Can you work these out from the model? Positions are in its coordinate system, mm. A direction names the side the tool comes from. Give positions to 0.01 mm unless a question says otherwise; leave off trailing zeros. Order: outer loops, then holes, each group sorted by start corner. A loop starts at its lowest first (then second) coordinate and runs counter-clockwise, first axis right, second up.
Item 1: I want a section at C-C, the plane y = 13. Write out the boundary of the cut face in (x, z), then the cut area to 3 significant figures.
Item 2: Which directions (+Z, -Z, +X, -X, +Y, -Y) give clear straight access to the entire face, cutting with the end or side of a thin tool? Please do faces 1 (the flat face through (-53.272, 10, 1)), 2 (the flat face through (38.836, 9.86, 25.136)), 3 (the flat face through (40.712, 9.86, 19.134)), 4 (the flat face through (37.063, 10, -23)).
Item 3: I'm going to push flat-ended pins straight in: pin 1 Ø3 at (y, z) = (12.5, -13.5) entering from -X; pin 2 Ø1.5 at (y, z) = (8.5, 11) entering from +X; pin 3 Ø5 at (y, z) = (9, 20.5) entering from +X. Where does each tip first touch, or does it pass through?
Item 4: If I drill on line 1 along Z through (x, y) = (42, 8.75); line 2 along Z through (x, y) = (41.5, 3); line 3 along X through (y, z) = (8.25, -2), over which ranges is the centre line in solid material (lowest first)?
Item 5: I want a section at B-B, the plane z = -20.5. Write out the boundary of the cut face in (x, y), then the cut area to 3 significant figures.
Item 6: If we mould it in two halves opening along Z, with no side actions, what happens to faces 5 (the flat face through (-11, 10, -27.075)), 6 (the cylindrical face through (43.73, 3.56, -19.28)), 7 (the flat face through (-58.473, 10, 24))? For each: +Z half, -Z half, draft (parallel to the pull), parting line (faces both ways), or undercut.
Item 7: I want a section at D-D, the plane z = -14. Write out the boundary of the cut face in (x, y), then the cut area to 3 significant figures.
Item 8: I want a section at A-A, the plane y = 6.5. Write out the boundary of the cut face in (x, z).
```python
from build123d import *

# Parameters (mm, degrees)
BOSS_EXTRUDE1_DEPTH = 20
SKETCH2_R           = 8.762238692
BOSS_EXTRUDE2_DEPTH = 13.528179
SKETCH3_W           = 5.200821941
SKETCH3_H           = 33.128455843
CUT_EXTRUDE1_DEPTH  = 69.647143148


with BuildPart() as part:
    # Sketch1 → Boss-Extrude1 (new body)
    with BuildSketch(Plane(origin=(0, 0, 0), x_dir=(1, 0, 0), z_dir=(0, 1, 0))):
        Polygon((37.062970991, 27.075407166), (37.062970991, 0.732918261), (31.104831338, -15.636935896), (50.591147993, -22.729375134), (48.442612656, -28.632427455), (28.956296002, -21.539988217), (25.917709331, -29.888436482), (-58.473170148, -29.888436482), (-58.473170148, 27.075407166), align=None)
    extrude(amount=BOSS_EXTRUDE1_DEPTH)

    # Sketch2 → Boss-Extrude2 (add)
    with BuildSketch(Plane(origin=(37.062970991, 0, 0), x_dir=(0, 0, -1), z_dir=(1, 0, 0))):
        with Locations(Location((12.821734178, 9.480390425, 0), (0, 0, 180))):
            Circle(SKETCH2_R)
    extrude(amount=BOSS_EXTRUDE2_DEPTH)

    # Sketch3 → Cut-Extrude1 (cut, through all)
    with BuildSketch(Plane(origin=(0, 20, 0), x_dir=(1, 0, 0), z_dir=(0, 1, 0))):
        with Locations((-55.872759178, -0.563117172)):
            Rectangle(SKETCH3_W, SKETCH3_H)
    extrude(amount=-CUT_EXTRUDE1_DEPTH, mode=Mode.SUBTRACT)


solid = part.part
```
Results list:
1. outline: (-58.47, -27.08) - (37.06, -27.08) - (37.06, -20.85) - (50.59, -20.85) - (50.59, -4.8) - (37.06, -4.8) - (37.06, -0.73) - (31.1, 15.64) - (50.59, 22.73) - (48.44, 28.63) - (28.96, 21.54) - (25.92, 29.89) - (-58.47, 29.89) - (-58.47, 17.13) - (-53.27, 17.13) - (-53.27, -16) - (-58.47, -16) - close
1. area: 5,450 mm2
2. face 1: -X, +Y, -Y
2. face 2: +Z, +Y, -Y
2. face 3: +X, +Y, -Y
2. face 4: +X
3. pin 1: stops at x = -53.27
3. pin 2: stops at x = 33.07
3. pin 3: stops at x = 50.59
4. line 1: z = -21.55 to -4.09, 19.6 to 26.29
4. line 2: z = -18.72 to -6.92, 19.42 to 26.11
4. line 3: x = -53.27 to 37.06
5. outline: (-58.47, 0) - (37.06, 0) - (37.06, 5.26) - (50.59, 5.26) - (50.59, 13.7) - (37.06, 13.7) - (37.06, 20) - (-58.47, 20) - close
5. area: 2,020 mm2
6. face 5: -Z half
6. face 6: undercut
6. face 7: draft
7. outline: (-53.27, 0) - (37.06, 0) - (37.06, 0.8) - (50.59, 0.8) - (50.59, 18.16) - (37.06, 18.16) - (37.06, 20) - (-53.27, 20) - close
7. area: 2,040 mm2
8. outline: (-58.47, -27.08) - (37.06, -27.08) - (37.06, -21.06) - (50.59, -21.06) - (50.59, -4.58) - (37.06, -4.58) - (37.06, -0.73) - (31.1, 15.64) - (50.59, 22.73) - (48.44, 28.63) - (28.96, 21.54) - (25.92, 29.89) - (-58.47, 29.89) - (-58.47, 17.13) - (-53.27, 17.13) - (-53.27, -16) - (-58.47, -16) - close
